```python
from build123d import *

# Parameters (mm, degrees)
F2_W     = 56.873322
F2_H     = 216.114152
F3_DEPTH = 58.238477


with BuildPart() as f1:
    # F0 (on Right) → F1 (revolve)
    with BuildSketch(Plane.YZ):
        with BuildLine():
            Line((-32.792136, 128.862843), (-36.590981, -0.143324))
            ThreePointArc((-36.590981, -0.143324), (-28.436845, -21.601239), (-7.5, -31.012967))
            ThreePointArc((-7.5, -31.012967), (-3.794939, -30.09838), (0, -29.695416))
            Line((0, -29.695416), (0, -29.452069))
            ThreePointArc((0, -29.452069), (-3.784372, -29.687502), (-7.485066, -30.51319))
            ThreePointArc((-7.485066, -30.51319), (-28.072963, -21.258324), (-36.091198, -0.158041))
            Line((-36.091198, -0.158041), (-32.292353, 128.848126))
            ThreePointArc((-32.292353, 128.848126), (-30.80293, 133.934638), (-27.016835, 137.64361))
            ThreePointArc((-27.016835, 137.64361), (-26.774217, 137.790861), (-26.539517, 137.950431))
            ThreePointArc((-26.539517, 137.950431), (-25.093616, 139.267941), (-23.989586, 140.882743))
            ThreePointArc((-23.989586, 140.882743), (-23.470074, 142.339477), (-23.376667, 143.883252))
            ThreePointArc((-23.376667, 143.883252), (-22.951827, 145.095666), (-22.810119, 146.372519))
            Line((-22.810119, 146.372519), (-23.310117, 146.371157))
            ThreePointArc((-23.310117, 146.371157), (-23.404957, 145.369883), (-23.691358, 144.405768))
            ThreePointArc((-23.691358, 144.405768), (-23.832133, 144.078405), (-23.86684, 143.723751))
            ThreePointArc((-23.86684, 143.723751), (-23.972267, 142.381072), (-24.432241, 141.115243))
            ThreePointArc((-24.432241, 141.115243), (-25.470912, 139.596038), (-26.831216, 138.356524))
            ThreePointArc((-26.831216, 138.356524), (-27.04458, 138.21146), (-27.265142, 138.077596))
            ThreePointArc((-27.265142, 138.077596), (-31.231715, 134.191822), (-32.792136, 128.862843))
        make_face()
    revolve(axis=Axis((0, 0, 66.14905), (0, 0, 1)))

    # F2 (on Right) → F3 (cut)
    with BuildSketch(Plane.YZ):
        with Locations((28.436661, 58.634361)):
            Rectangle(F2_W, F2_H)
    extrude(amount=-F3_DEPTH, mode=Mode.SUBTRACT)


solid = f1.part
```
The model under review builds one solid part; all positions refer to its coordinate system, in mm. Round coordinates to 2 decimals unless told otherwise and drop trailing zeros. Loops run counter-clockwise (first coordinate to the right, second up) from the corner with the lowest first, then second, coordinate; pieces in that order, holes last. Notation, with made-up numbers: (12, 17) - (17, 17) arc R18 ccw to (17, 27) - close; hole circle Ø9 at (24, 12). An arc over 180 degrees is marked (long way). Write each question's results on one line, items separated by ' | '. Start each with the question number.
Q1. Take a section at A-A on z = 35.5. Give the boundary of the cut face in (x, y), plus the area to 3 significant figures.
Q2. Take a section at B-B on z = 102. Give the boundary of the cut face in (x, y).
Q3. Insertion check: P1, Ø5, axis at x = -6, z = 51, coming from the +Y side; P2, Ø10, axis at x = -28.5, z = 64.5, coming from the -Y side; P3, Ø2, axis at y = 22.5, z = 3.5, coming from the +X side. Each pin has a flat end and moves straight along its axis. Give the tip position at first contact, or say it passes through.
Q4. Wall thickness on line 1 along Z through (x, y) = (23, 16); line 2 along Y through (x, z) = (4, 115); line 3 along Y through (x, z) = (19, 32.5): over which ranges is each line inside the solid? List them lowest first. Write a range as [from, to].
Q5. Draft analysis for pull direction X (two halves, no side actions). For faces 1 (the conical face through (23.35, -24.94, 65.25)), 2 (the conical face through (23.726, -25.346, 63.457)), state which applies: pulls with the +X half, pulls with the -X half, needs draft (parallel to the pull), parting line crosses it, or undercut.
Data:
1) outline: (-35.54, 0) arc R35.54 ccw (long way) to (0, 35.54) - (0, 35.04) arc R35.04 cw (long way) to (-35.04, 0) - close | area: 83.2 mm²
2) outline: (-33.58, 0) arc R33.58 ccw (long way) to (0, 33.58) - (0, 33.08) arc R33.08 cw (long way) to (-33.08, 0) - close
3) P1: stops at y = -33.52 | P2: stops at y = -25.52 | P3: stops at x = 29.48
4) line 1: z = [-22.04, -21.32], [136.99, 137.61] | line 2: y = [-32.96, -32.45], [32.45, 32.96] | line 3: y = [-30.14, -29.55], [29.55, 30.14]
5) face 1: undercut | face 2: parting line crosses it
